Could you check a few things on this model? Use its own coordinates, in mm. Face numbers are marked on the shaded views. A direction names the side the tool comes from. Coordinates: 2 decimals unless noted, no trailing zeros. Order: outer loops, then holes, each group sorted by start corner. A loop starts at its lowest first (then second) coordinate and runs counter-clockwise, first axis right, second up. Notation, with made-up numbers: (83.5, 87.25) - (128.5, 87.25) arc R19 ccw to (128.5, 107.25) - close; hole circle Ø5 at (65.5, -9). An arc over 180 degrees is marked (long way). One line per item, written item: value.
from build123d import *

# Parameters (mm, degrees)
REVOLVE1_ANGLE     = 45
CUT_REVOLVE5_ANGLE = 23
SKETCH5_R          = 2.5
CUT_EXTRUDE1_DEPTH = 2.55


with BuildPart() as part:
    # Sketch1 → Revolve1 (revolve, symmetric)
    with BuildSketch(Plane.XY) as revolve1_sk:
        with BuildLine():
            Line((-26.239989701, -17.447458038), (-26.239989701, -0.731138339))
            ThreePointArc((-26.239989701, -0.731138339), (-25.865330741, 2.115285345), (-24.766875558, 4.767811185))
            Line((-24.766875558, 4.767811185), (-20.234178791, 12.620671907))
            ThreePointArc((-20.234178791, 12.620671907), (-19.135723608, 15.273197747), (-18.761064648, 18.119621431))
            Line((-18.761064648, 18.119621431), (-18.761064648, 20.793898522))
            Line((-18.761064648, 20.793898522), (-8.983798531, 20.825060578))
            Line((-8.983798531, 20.825060578), (-8.983798531, 10.405785055))
            ThreePointArc((-8.983798531, 10.405785055), (-11.144661105, 8.19078498), (-12.908903509, 5.648541651))
            Line((-12.908903509, 5.648541651), (-26.239989701, -17.447458038))
        make_face()
    revolve(axis=Axis((0, 0, 0), (0, -1, 0)), revolution_arc=REVOLVE1_ANGLE / 2)
    revolve(revolve1_sk.sketch, axis=Axis((0, 0, 0), (0, 1, 0)), revolution_arc=REVOLVE1_ANGLE / 2)

    # Sketch4 → Cut-Revolve5 (revolve, symmetric, cut)
    with BuildSketch(Plane.XY) as cut_revolve5_sk:
        with BuildLine():
            Line((-18.06897746, 11.370910651), (-22.601674227, 3.51804993))
            ThreePointArc((-22.601674227, 3.51804993), (-23.450480505, 1.468370871), (-23.739989701, -0.731138339))
            Line((-23.739989701, -0.731138339), (-23.739989701, -8.115272969))
            Line((-23.739989701, -8.115272969), (-15.07410484, 6.898302907))
            ThreePointArc((-15.07410484, 6.898302907), (-13.438873503, 9.325699255), (-11.483798531, 11.503752607))
            Line((-11.483798531, 11.503752607), (-11.483798531, 18.317079893))
            Line((-11.483798531, 18.317079893), (-16.261064648, 18.301853813))
            Line((-16.261064648, 18.301853813), (-16.261064648, 18.119621431))
            ThreePointArc((-16.261064648, 18.119621431), (-16.720873371, 14.626283274), (-18.06897746, 11.370910651))
        make_face()
    revolve(axis=Axis((0, 0, 0), (0, -1, 0)), revolution_arc=CUT_REVOLVE5_ANGLE / 2, mode=Mode.SUBTRACT)
    revolve(cut_revolve5_sk.sketch, axis=Axis((0, 0, 0), (0, 1, 0)), revolution_arc=CUT_REVOLVE5_ANGLE / 2, mode=Mode.SUBTRACT)

    # Sketch5 → Cut-Extrude1 (cut)
    with BuildSketch(Plane(origin=(-0.071940118, 20.85344552, 0), x_dir=(-0.9999940495093123, -0.003449774770501149, 0), z_dir=(0.003449774770501149, -0.9999940495093123, 0))):
        with Locations(Location((13.8, 0, 0), (0, 0, 342.175900363))):
            Circle(SKETCH5_R)
    extrude(amount=CUT_EXTRUDE1_DEPTH, mode=Mode.SUBTRACT)


solid = part.part
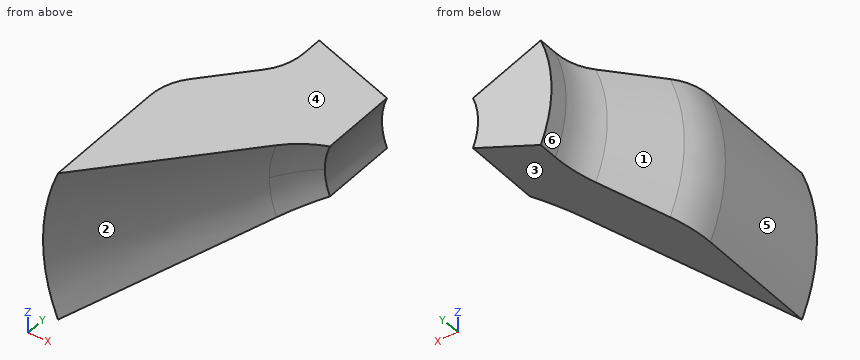
Item 1: I want a section at C-C on y = -10.5. Please give me the cut outline in (x, z).
Conclusion:
outline: (-24.24, -10.04) - (-20.54, -8.51) arc R22.23 cw to (-20.54, 8.51) - (-24.24, 10.04) arc R26.24 ccw to start
Item 2: I'm going to push flat-ended pins straight in: pin 1 Ø10 at (y, z) = (-1.5, 5) entering from +X; pin 2 Ø10 at (x, z) = (-14, 0.5) entering from -Y; pin 3 Ø5 at (x, y) = (-15.5, 14) entering from -Z. Where does each tip first touch, or does it pass through?
Conclusion:
pin 1: x = -13.08
pin 2: y = -4.92
pin 3: z = -7.46
Item 3: Thinking about a two-plate mould opening in Z: for the marked faces 1, 2, 3 and 4, which applies, pulls with the +Z half, pulls with the -Z half, needs draft (parallel to the pull), parting line crosses it, or undercut?
Conclusion:
face 1: parting line crosses it
face 2: undercut
face 3: pulls with the -Z half
face 4: pulls with the +Z half
Item 4: I want a section at A-A on y = -2. Please give me the cut outline in (x, z).
Conclusion:
outline: (-24.24, -10.04) - (-16, -6.63) arc R17.32 cw to (-16, 6.63) - (-24.24, 10.04) arc R26.24 ccw to start; hole (-23.26, -4.73) - (-19.8, -4.03) arc R20.21 cw to (-19.8, 4.03) - (-23.26, 4.73) arc R23.74 ccw to start
Item 5: I want a section at B-B on y = 12. Please give me the cut outline in (x, z).
Conclusion:
outline: (-19.02, -7.88) - (-8.3, -3.44) arc R8.98 cw to (-8.3, 3.44) - (-19.02, 7.88) arc R20.59 ccw to start; hole (-17.37, -3.53) - (-11.25, -2.29) arc R11.48 cw to (-11.25, 2.29) - (-17.37, 3.53) arc R17.73 ccw to start
Item 6: If I drill on probe 1 along Z at (x, y) = (-21.25, 0); probe 2 along X at (y, z) = (3, -2.5); probe 3 along Y at (x, z) = (-18, 2.5), over which ranges is the centre line in solid material (lowest first)?
Conclusion:
probe 1: -8.8 to -4.32, 4.32 to 8.8
probe 2: -25.47 to -22.74, -17.14 to -14.22
probe 3: -3.47 to 1.53, 11.19 to 20.8
Item 7: For the marked faces 5 and 6, which set-ups out of +Z, -Z, +X, -X, +Y, -Y let a thin tool reach every point of the face, with its end or its side?
Conclusion:
face 5: -X, +Y, -Y
face 6: -X, +Y
